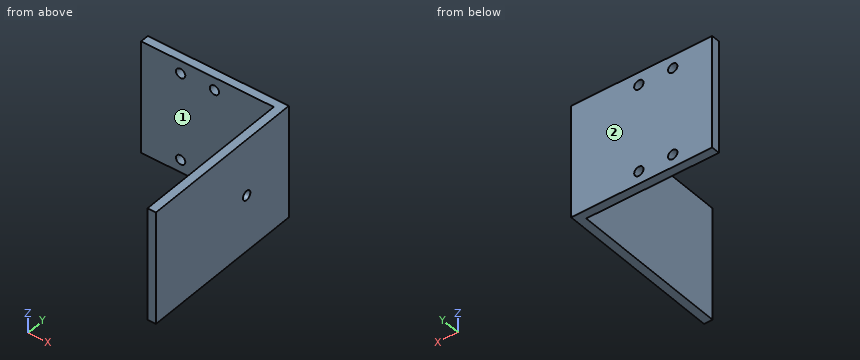
```python
from build123d import *

# Parameters (mm, degrees)
EXTRUDE_1_DEPTH     = 40
SKETCH_2_R          = 1.65
CUT_EXTRUDE_1_DEPTH = 10
SKETCH_3_R          = 1.65
CUT_EXTRUDE_2_DEPTH = 10


with BuildPart() as part:
    # 草图1 → 凸台-拉伸1 (new body)
    with BuildSketch(Plane.XY):
        Polygon((0, 0), (50, 0), (50, -60), (47, -60), (47, -3), (0, -3), align=None)
    extrude(amount=EXTRUDE_1_DEPTH)

    # 草图2 → 切除-拉伸1 (cut)
    with BuildSketch(Plane(origin=(0, 0, 0), x_dir=(1, 0, 0), z_dir=(0, 1, 0))):
        with Locations((14, -4.5)):
            Circle(SKETCH_2_R)
        with Locations((14, -35.5)):
            Circle(SKETCH_2_R)
        with Locations((26, -4.5)):
            Circle(SKETCH_2_R)
        with Locations((26, -35.5)):
            Circle(SKETCH_2_R)
    extrude(amount=-CUT_EXTRUDE_1_DEPTH, mode=Mode.SUBTRACT)

    # 草图3 → 切除-拉伸2 (cut)
    with BuildSketch(Plane(origin=(50, 0, 0), x_dir=(0, 0, -1), z_dir=(1, 0, 0))):
        with Locations((-20, -19.05)):
            Circle(SKETCH_3_R)
    extrude(amount=-CUT_EXTRUDE_2_DEPTH, mode=Mode.SUBTRACT)


solid = part.part
```
The model under review builds one solid part; all positions refer to its coordinate system, in mm. Face numbers are marked on the shaded views. A direction names the side the tool comes from. Coordinates: 2 decimals unless noted, no trailing zeros. Loops run counter-clockwise (first coordinate to the right, second up) from the corner with the lowest first, then second, coordinate; pieces in that order, holes last. Notation, with made-up numbers: (-18.5, -13) -> (-7.5, -13) arc R14 cw to (-7.5, -8) -> close; hole circle Ø2 at (5, 34). An arc over 180 degrees is marked (long way). Answer as CSV lines item,"result".
Item 1: Machinability: for the marked faces 1 and 2, which of the approach directions +Z, -Z, +X, -X, +Y, -Y give a long, thin tool a straight path to every point of the face, cutting with its end or side? Answer none if there is none.
Results below:
face 1,"+Z, -Z, -X, -Y"
face 2,"+Z, -Z, +X, -X, +Y"
Item 2: Take a section at D-D, the plane x = 43. State the section outline as (y, z) points.
Results below:
outline,"(-3, 0) -> (0, 0) -> (0, 40) -> (-3, 40) -> close"
Item 3: Take a section at C-C, the plane z = 35.5. State the section outline as (x, y) points.
Results below:
outline,"(0, -3) -> (12.35, -3) -> (12.35, 0) -> (0, 0) -> close; (15.65, -3) -> (24.35, -3) -> (24.35, 0) -> (15.65, 0) -> close; (27.65, -3) -> (47, -3) -> (47, -60) -> (50, -60) -> (50, 0) -> (27.65, 0) -> close"
Item 4: Take a section at B-B, the plane x = 26. State the section outline as (y, z) points.
Results below:
outline,"(-3, 0) -> (0, 0) -> (0, 2.85) -> (-3, 2.85) -> close; (-3, 6.15) -> (0, 6.15) -> (0, 33.85) -> (-3, 33.85) -> close; (-3, 37.15) -> (0, 37.15) -> (0, 40) -> (-3, 40) -> close"
Item 5: Insertion check: pin 1 (6 mm diameter, centred on x = 11, z = 16.5, fed in from -Y); pin 2 (3 mm diameter, centred on y = -19.05, z = 20, fed in from -X) (1 decimal); pin 3 (10 mm diameter, centred on y = -52, z = 11, fed in from -X). Each pin has a flat end and moves straight along its axis. Give the tip position at first contact, or say it passes through.
Results below:
pin 1,"stops at y = -3"
pin 2,"passes through"
pin 3,"stops at x = 47"
Item 6: Take a section at A-A, the plane z = 20. State the section outline as (x, y) points, and give its area (3 significant figures).
Results below:
outline,"(0, -3) -> (47, -3) -> (47, -17.4) -> (50, -17.4) -> (50, 0) -> (0, 0) -> close; (47, -60) -> (50, -60) -> (50, -20.7) -> (47, -20.7) -> close"
area,"311 mm2"
Item 7: For L1, parallel to Z at x = 26, y = -0.9; L2, parallel to X at y = -2.15, z = 4.5; L3, parallel to Y at x = 48.4, z = 20, list the stretches that pass through material, from the lowest coordinate up.
Results below:
L1,"z = 0 to 2.85, 6.15 to 33.85, 37.15 to 40"
L2,"x = 0 to 12.35, 15.65 to 24.35, 27.65 to 50"
L3,"y = -60 to -20.7, -17.4 to 0"
